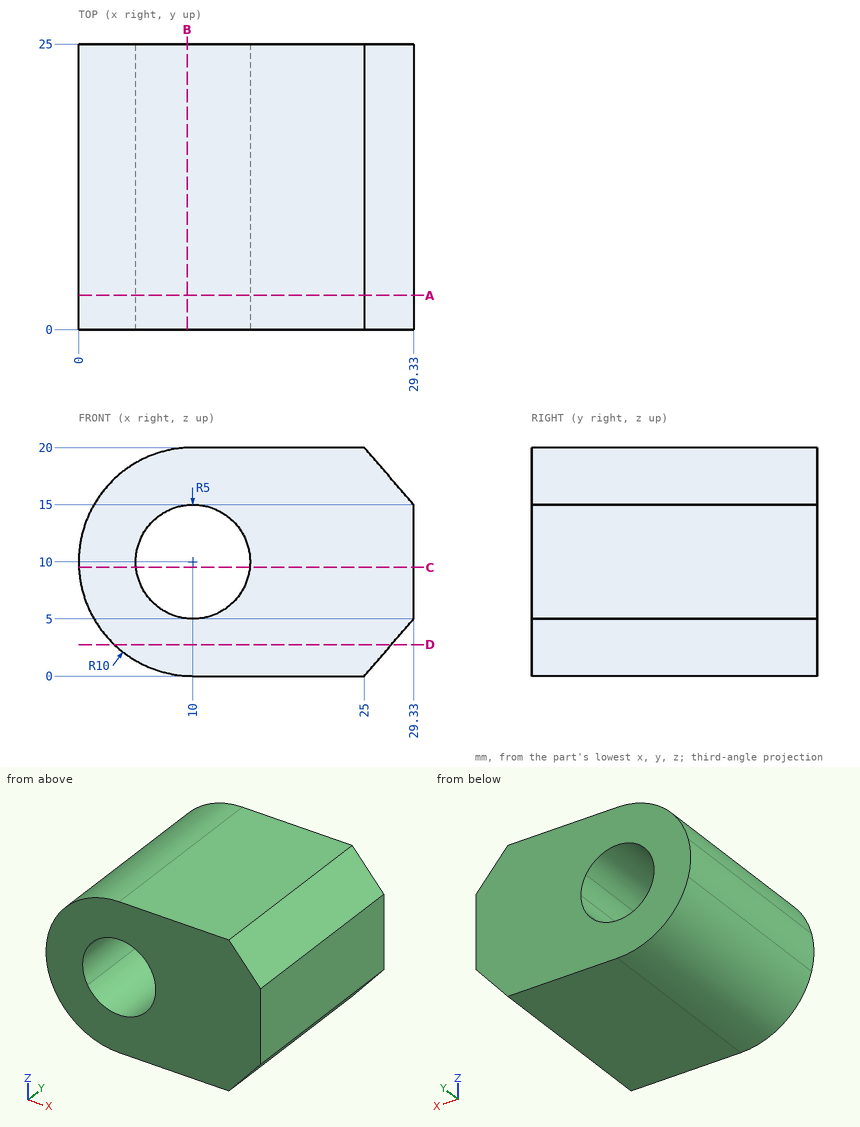
Could you check a few things on this drawing? It's one solid part, dimensions in mm from its lowest x, y, z. Round coordinates to 2 decimals unless told otherwise and drop trailing zeros. Loops run counter-clockwise (first coordinate to the right, second up) from the corner with the lowest first, then second, coordinate; pieces in that order, holes last. Notation, with made-up numbers: (20, 77) -> (37, 77) arc R16 cw to (37, 87) -> close; hole circle Ø9 at (28, 0). An arc over 180 degrees is marked (long way). Write each question's results on one line, items separated by ' | '.
(1) If we section it at C-C, the plane z = 9.5: List the corners of the cut face in (x, y) for me (1 decimal).
Worked answers:
outline: (0, 0) -> (5, 0) -> (5, 25) -> (0, 25) -> close; (15, 0) -> (29.3, 0) -> (29.3, 25) -> (15, 25) -> close
(2) If we section it at A-A, the plane y = 3: List the corners of the cut face in (x, z) for me, then the cut area to 4 significant figures.
Worked answers:
outline: (0.32, 7.5) arc R10 ccw to (10, 0) -> (25, 0) -> (29.33, 5) -> (29.33, 15) -> (25, 20) -> (10, 20) arc R10 ccw to (0.32, 12.5) arc R10 ccw to start; hole (14.33, 7.5) arc R5 ccw to (15, 10) arc R5 ccw to (14.33, 12.5) arc R5 ccw (long way) to start | area: 443.5 mm2
(3) For P1, Ø6, axis at x = 5.5, y = 21.5, coming from the +Z side, with a flat end and sliding along its axis, tell me the tip position at first contact or that it passes through.
Worked answers:
P1: z = 19.89
(4) If we section it at B-B, the plane x = 9.5: List the corners of the cut face in (y, z) for me (1 decimal), then the cut area to 3 significant figures.
Worked answers:
outline: (0, 0) -> (25, 0) -> (25, 5) -> (0, 5) -> close; (0, 15) -> (25, 15) -> (25, 20) -> (0, 20) -> close | area: 251 mm2
(5) If we section it at D-D, the plane z = 2.75: List the corners of the cut face in (x, y) for me.
Worked answers:
outline: (3.11, 0) -> (27.38, 0) -> (27.38, 25) -> (3.11, 25) -> close
(6) If I drill on L1, parallel to X at y = 10.25, z = 12.5; L2, parallel to Z at x = 10, y = 4.75; L3, parallel to Z at x = 8.5, y = 15.75, over which ranges is the centre line in solid material (lowest first)?
Worked answers:
L1: 0.32 to 5.67, 14.33 to 29.33 | L2: 0 to 5, 15 to 20 | L3: 0.11 to 5.23, 14.77 to 19.89
